Autodesk Inventor part; units mm, degrees
ref_plane "YZ Plane" through (0, 0, 0) normal (1, 0, 0) x (0, 1, 0)
ref_plane "XZ Plane" through (0, 0, 0) normal (0, 1, 0) x (-1, 0, 0)
ref_plane "XY Plane" through (0, 0, 0) normal (0, 0, 1) x (1, 0, 0)
sketch "Sketch8" plane through (0, 0, 0) normal (0, 1, 0) x (-1, 0, 0)
  line L0 (-65.5, -64.5) -> (65.5, -64.5)
  line L1 (65.5, -64.5) -> (65.5, 64.5)
  line L2 (65.5, 64.5) -> (-65.5, 64.5)
  line L3 (-65.5, 64.5) -> (-65.5, -64.5)
  line L4 (-65.5, -64.5) -> (65.5, 64.5) construction
  line L5 (65.5, -64.5) -> (-65.5, 64.5) construction
  point P0 (0, 0)
  dimension "d26" = 131
  dimension "d27" = 129
extrude "Extrusion7" add sketch "Sketch8" along normal blind 95
sketch "Sketch9" plane through (0, 0, 0) normal (0, -1, 0) x (1, 0, 0)
  line L0 (-65.5, 64.5) -> (65.5, 64.5)
  line L1 (-65.5, -64.5) -> (65.5, -64.5)
  line L2 (65.5, -64.5) -> (65.5, 64.5)
  line L3 (65.5, 64.5) -> (-65.5, 64.5)
  line L4 (-65.5, 64.5) -> (-65.5, -64.5)
  line L5 (-65.5, -64.5) -> (65.5, 64.5) construction
  line L6 (65.5, -64.5) -> (-65.5, 64.5) construction
  line L7 (61.5, 60.5) -> (61.5, -60.5)
  line L8 (61.5, -60.5) -> (-65.5, -60.5)
  line L9 (-65.5, 60.5) -> (61.5, 60.5)
  line L10 (57.5, -56.5) -> (57.5, 56.5)
  line L11 (57.5, 56.5) -> (-65.5, 56.5)
  line L12 (-65.5, -56.5) -> (57.5, -56.5)
  line L13 (-63.4537, -60.5) -> (-63.4537, -62.485)
  line L14 (-63.4537, 62.485) -> (-63.4537, 60.5)
  line L15 (-59.3922, 56.5) -> (-59.3922, 58.4854)
  line L16 (-59.3922, -58.4854) -> (-59.3922, -56.5)
  point P0 (0, 0)
  dimension "d30" = 4
  dimension "d31" = 4
  dimension "d47" = 4
  dimension "d48" = 4
  dimension "d49" = 4
  dimension "d50" = 4
extrude "Extrusion8" cut sketch "Sketch9" against normal blind 115 contours L11 L10 L12 L4
extrude "Extrusion9" cut sketch "Sketch9" against normal blind 90 contours L9 L7 L8 L4 L12 L10 L11
sketch "Sketch10" plane through (0, 0, 0) normal (0, -1, 0) x (1, 0, 0)
  line L0 (65.5, -64.5) -> (-65.5, -64.5)
  line L1 (-65.5, -64.5) -> (-65.5, 64.5)
  line L2 (-65.5, 64.5) -> (65.5, 64.5)
  line L3 (65.5, 64.5) -> (65.5, -64.5)
  line L4 (65.5, -64.5) -> (-65.5, 64.5) construction
  line L5 (-65.5, -64.5) -> (65.5, 64.5) construction
  line L6 (-69.5, 68.5) -> (-69.5, -68.5)
  line L7 (-69.5, -68.5) -> (69.5, -68.5)
  line L8 (69.5, -68.5) -> (69.5, 68.5)
  line L9 (69.5, 68.5) -> (-69.5, 68.5)
  line L10 (-65.5, 64.5) -> (-69.5, 64.5)
  line L11 (-65.5, -64.5) -> (-69.5, -64.5)
  line L12 (-65.5, 64.5) -> (-65.5, 68.5)
  line L13 (-65.5, -64.5) -> (-65.5, -68.5)
  point P0 (0, 0)
  dimension "d36" = 4
extrude "Extrusion10" add sketch "Sketch10" against normal blind 5 contours L3 L2 L12 L9 L8 L7 L13 L0
sketch "Sketch11" plane through (0, 0, 0) normal (0, -1, 0) x (1, 0, 0)
  circle A0 centre (-66.5, 0.5) radius 135
  line L0 (61.5, 60.5) -> (61.5, -60.5)
  line L1 (69.5, -68.5) -> (69.5, 68.5)
  circle A1 centre (-66.5, 0.5) radius 110
  line L2 (19.168, -68.5) -> (69.5, -68.5)
  line L3 (69.5, -68.5) -> (69.5, 68.5)
  line L4 (69.5, 68.5) -> (19.9639, 68.5)
  line L5 (-65.5, 68.5) -> (69.5, 68.5)
  point P0 (0, 0)
  dimension "d39" = 270
  dimension "d41" = 136
  dimension "d42" = 220
extrude "Extrusion11" cut sketch "Sketch11" against normal blind 1.125 contours A0 L0 | A0 L4 L1 L2 | L0 A0 L2 A1 L4
properties part number "Galvo Housing-01"
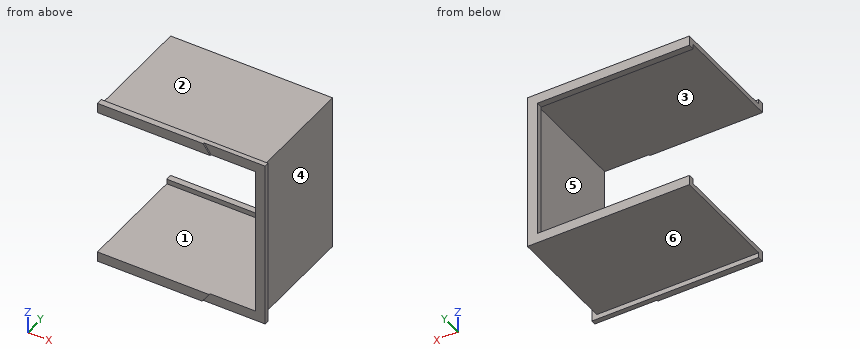
Source: CAD feature listing. Evaluate the final solid. Frame: model axes, mm. Face numbers are marked on the shaded views. A direction names the side the tool comes from. Round coordinates to 2 decimals unless told otherwise and drop trailing zeros. Loops run counter-clockwise (first coordinate to the right, second up) from the corner with the lowest first, then second, coordinate; pieces in that order, holes last. Notation, with made-up numbers: M 86.5,36.25 L 143.5,36.25 A7 ccw 143.5,47.25 Z; hole C -1.5,-17.5 d11. An arc over 180 degrees is marked long. Return JSON: item names as keys, results as strings. Group by question number.
1. Section query B-B on y = 42. Output: boundary loops of the cut face in (x, z), and give its area (3 significant figures).
2. Material intervals for line 1 along Z through (x, y) = (-47, 29); line 2 along X through (y, z) = (28.5, -2); line 3 along Y through (x, z) = (62, -12) (3 decimals), sorted ascending. Write a range as from..to.
3. Section query C-C on z = -27.5. Output: boundary loops of the cut face in (x, y) (3 decimals).
4. Pin query (flat end, axial travel): pin 1 (4 mm diameter, centred on y = 93.5, z = 24, fed in from -X); pin 2 (6 mm diameter, centred on x = -17.5, y = 64.5, fed in from -Z); pin 3 (12 mm diameter, centred on y = 56.5, z = -2.5, fed in from -X). Return the tip coordinate at first contact, or that it passes through.
5. Reachability of the marked faces 1 and 2 from +Z, -Z, +X, -X, +Y, -Y: full face, straight path, thin tool, end or side. Return the list, or none.
6. Section query A-A on x = -40.5. Output: boundary loops of the cut face in (y, z).
7. Mould query, pull axis Z, two halves, no side actions, for the marked faces 3, 4, 5 and 6. Classes: released by +Z, released by -Z, zero draft, split by the parting line, or undercut.
Checks:
{
 "1": {"outline": "M -65.5,-64.5 L 65.5,-64.5 L 65.5,64.5 L -65.5,64.5 L -65.5,60.5 L 61.5,60.5 L 61.5,-60.5 L -65.5,-60.5 Z", "area": "1,530 mm²"},
 "2": {"line 1": "z = -64.5..-60.5, 60.5..64.5", "line 2": "x = 61.5..65.5", "line 3": "y = 1.125..95"},
 "3": {"outline": "M 57.5,90 L 61.5,90 L 61.5,1.125 L 69.5,1.125 L 69.5,5 L 65.5,5 L 65.5,95 L 57.5,95 Z"},
 "4": {"pin 1": "stops at x = 57.5", "pin 2": "stops at z = -64.5", "pin 3": "stops at x = 61.5"},
 "5": {"face 1": "-X, -Y", "face 2": "+Z, +X, -X, +Y"},
 "6": {"outline": "M 0,-68.5 L 5,-68.5 L 5,-64.5 L 95,-64.5 L 95,-56.5 L 90,-56.5 L 90,-60.5 L 0,-60.5 Z; M 0,60.5 L 90,60.5 L 90,56.5 L 95,56.5 L 95,64.5 L 5,64.5 L 5,68.5 L 0,68.5 Z"},
 "7": {"face 3": "undercut", "face 4": "zero draft", "face 5": "undercut", "face 6": "released by -Z"}
}
